```python
from build123d import *

# Parameters (mm, degrees)
SKETCH1_W                  = 44.45
SKETCH1_H                  = 22.86
SKETCH1_R                  = 4.7625
BOSS_EXTRUDE1_DEPTH        = 7.62
F_6_32_TAPPED_HOLE1_REACH  = 34.781
F_6_32_TAPPED_HOLE1_BORE_R = 1.35255
CUT_EXTRUDE2_REACH         = 28.128
SKETCH19_W                 = 12.7
SKETCH19_H                 = 19.05
F_6_CLEARANCE_HOLE1_D      = 3.7973
SKETCH24_W                 = 2.54
SKETCH24_H                 = 7.62
BOSS_EXTRUDE2_DEPTH        = 10.16
F_6_32_TAPPED_HOLE5_D      = 2.7051


with BuildPart() as part:
    # Sketch1 → Boss-Extrude1 (new body)
    with BuildSketch(Plane(origin=(0, 0, 0), x_dir=(1, 0, 0), z_dir=(0, 1, 0))):
        Rectangle(SKETCH1_W, SKETCH1_H)
        with Locations(Location((0, 0, 0), (0, 0, 90))):
            Circle(SKETCH1_R, mode=Mode.SUBTRACT)
    extrude(amount=BOSS_EXTRUDE1_DEPTH)

    # #6-32 Tapped Hole1 bore → #6-32 Tapped Hole1 (cut, up to next)
    with BuildSketch(Plane(origin=(0, 0, -11.43), x_dir=(-1, 0, 0), z_dir=(0, 0, -1)), mode=Mode.PRIVATE) as f_6_32_tapped_hole1_sk1:
        with Locations((0, 3.81)):
            Circle(F_6_32_TAPPED_HOLE1_BORE_R)
    f_6_32_tapped_hole1_tool1 = extrude(f_6_32_tapped_hole1_sk1.sketch, amount=-F_6_32_TAPPED_HOLE1_REACH, mode=Mode.PRIVATE) & part.part
    add(f_6_32_tapped_hole1_tool1.solids().sort_by_distance((0, 3.81, -11.43))[0], mode=Mode.SUBTRACT)

    # Sketch19 → Cut-Extrude2 (cut, up to next)
    with BuildSketch(Plane(origin=(0, 7.62, 0), x_dir=(1, 0, 0), z_dir=(0, 1, 0)), mode=Mode.PRIVATE) as cut_extrude2_sk1:
        with Locations((-15.875, -1.905)):
            Rectangle(SKETCH19_W, SKETCH19_H)
    cut_extrude2_tool1 = extrude(cut_extrude2_sk1.sketch, amount=-CUT_EXTRUDE2_REACH, mode=Mode.PRIVATE) & part.part
    cut_extrude2 = cut_extrude2_tool1.solids().sort_by_distance((-15.875, 7.62, 1.905))[0]
    add(cut_extrude2, mode=Mode.SUBTRACT)

    # #6 Clearance Hole1 (through all)
    with Locations(Plane.XY.offset(-7.62)):
        with Locations((-14.605, 3.81)):
            f_6_clearance_hole1 = Hole(F_6_CLEARANCE_HOLE1_D / 2)

    # Mirror4: Cut-Extrude2, #6 Clearance Hole1 across plane
    add(cut_extrude2.mirror(Plane(origin=(0, 0, 0), x_dir=(0, 0, 1), z_dir=(1, 0, 0))), mode=Mode.SUBTRACT)
    add(f_6_clearance_hole1.mirror(Plane(origin=(0, 0, 0), x_dir=(0, 0, 1), z_dir=(1, 0, 0))), mode=Mode.SUBTRACT)

    # Sketch24 → Boss-Extrude2 (add)
    with BuildSketch(Plane.XY.offset(-7.62)):
        with Locations((-20.955, 3.81)):
            Rectangle(SKETCH24_W, SKETCH24_H)
    boss_extrude2 = extrude(amount=BOSS_EXTRUDE2_DEPTH)

    # Mirror5: Boss-Extrude2 across plane
    add(boss_extrude2.mirror(Plane(origin=(0, 0, 0), x_dir=(0, 0, 1), z_dir=(1, 0, 0))))

    # #6-32 Tapped Hole5 (through all)
    with Locations(Plane(origin=(0, 7.62, 0), x_dir=(1, 0, 0), z_dir=(0, 1, 0))):
        with Locations((-5.715, -7.62), (5.715, -7.62)):
            Hole(F_6_32_TAPPED_HOLE5_D / 2)


solid = part.part
```
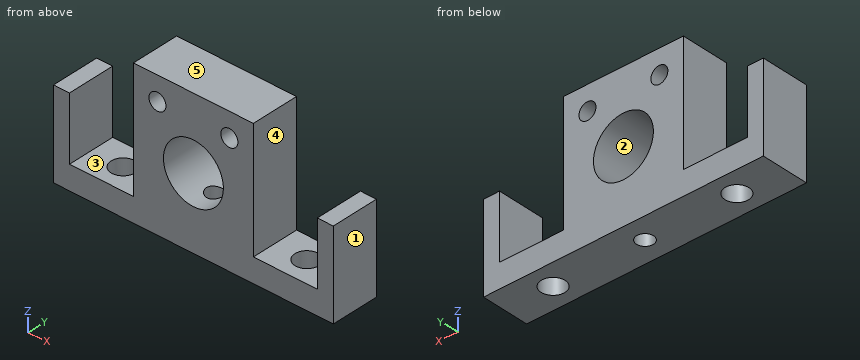
Model file for the job. Use its own axes, mm. Face numbers are marked on the shaded views. A direction names the side the tool comes from. Give positions to 0.01 mm unless a question says otherwise; leave off trailing zeros. Write each loop counter-clockwise with the first axis right and the second up, starting at its lowest first coordinate (ties: lowest second). Pieces come first, ordered by that corner, then holes. Notation, with made-up numbers: (84.5, 15.5) - (137.5, 15.5) arc R22 ccw to (137.5, 21.5) - close; hole circle Ø3 at (67, 19). An arc over 180 degrees is marked (long way). One line per question, with ' | ' between items. Start each with the question number.
(1) Two-plate mould, pull along Z, no slides. Class the marked faces 1, 2 and 3: +Z half, -Z half, draft (parallel to the pull), parting line (faces both ways), or undercut.
(2) 3-axis set-ups, long thin cutter, end or side, ignore diameter. For the marked faces 4 and 5: which of +Z, -Z, +X, -X, +Y, -Y reach the whole face in a straight line?
(3) Slice it at C-C on x = 0. Write the cut outline in (y, z).
(4) Slice it at D-D on z = 7.62. Write the cut outline in (x, y) (3 decimals), plus the area to 3 significant figures.
(5) Slice it at A-A on z = -6. Write the cut outline in (x, y) (3 decimals).
(6) Pin check, flat tips, straight feed: P1, Ø2.5, axis at x = -5.715, z = 7.62, coming from the +Y side; P2, Ø2, axis at x = -20.5, y = 2.5, coming from the +Z side; P3, Ø1, axis at y = 4, z = 5, coming from the +X side (3 decimals); P4, Ø4, axis at x = 12.5, y = 2, coming from the +Z side. Stop position of each tip, or through.
(7) Slice it at B-B on y = 3.81. Write the cut outline in (x, z) (1 decimal).
(8) Wall check: line 1 along X through (y, z) = (4.25, 7.62) (3 decimals); line 2 along X through (y, z) = (3.5, 0) (1 decimal); line 3 along X through (y, z) = (7.25, -6) (3 decimals). Give the ranges that are in metal, low to high. Write a range as from..to.
Results below:
1) face 1: draft | face 2: undercut | face 3: +Z half
2) face 4: +Z, +Y, -Y | face 5: +Z, +X, -X, +Y, -Y
3) outline: (0, -11.43) - (2.46, -11.43) - (2.46, -4.76) - (0, -4.76) - close; (0, 4.76) - (7.62, 4.76) - (7.62, 11.43) - (0, 11.43) - close; (5.16, -11.43) - (7.62, -11.43) - (7.62, -4.76) - (5.16, -4.76) - close
4) outline: (-9.525, 0) - (-7.068, 0) - (-7.068, 7.62) - (-9.525, 7.62) - close; (-4.362, 0) - (4.362, 0) - (4.362, 7.62) - (-4.362, 7.62) - close; (7.068, 0) - (9.525, 0) - (9.525, 7.62) - (7.068, 7.62) - close | area: 104 mm^2
5) outline: (-22.225, 0) - (-19.685, 0) - (-19.685, 7.62) - (-22.225, 7.62) - close; (-9.525, 0) - (9.525, 0) - (9.525, 7.62) - (-9.525, 7.62) - close; (19.685, 0) - (22.225, 0) - (22.225, 7.62) - (19.685, 7.62) - close; hole circle Ø2.705 at (0, 3.81)
6) P1: through | P2: z = 2.54 | P3: x = 9.525 | P4: z = -7.62
7) outline: (-22.2, -11.4) - (-16.5, -11.4) - (-16.5, -7.6) - (-19.7, -7.6) - (-19.7, 2.5) - (-22.2, 2.5) - close; (-12.7, -11.4) - (-1.4, -11.4) - (-1.4, -4.6) arc R4.8 cw (long way) to (1.4, -4.6) - (1.4, -11.4) - (12.7, -11.4) - (12.7, -7.6) - (9.5, -7.6) - (9.5, 11.4) - (-9.5, 11.4) - (-9.5, -7.6) - (-12.7, -7.6) - close; (16.5, -11.4) - (22.2, -11.4) - (22.2, 2.5) - (19.7, 2.5) - (19.7, -7.6) - (16.5, -7.6) - close; hole circle Ø2.7 at (-5.7, 7.6); hole circle Ø2.7 at (5.7, 7.6)
8) line 1: -9.525..-7.068, -4.362..4.362, 7.068..9.525 | line 2: -22.2..-19.7, -9.5..-4.8, 4.8..9.5, 19.7..22.2 | line 3: -22.225..-19.685, -9.525..9.525, 19.685..22.225
